from build123d import *

# Parameters (mm, degrees)
SKETCH1_W           = 12
SKETCH1_H           = 18.3
BOSS_EXTRUDE1_DEPTH = 3
SKETCH2_W           = 6
SKETCH2_H           = 18.3
BOSS_EXTRUDE2_DEPTH = 6
SKETCH3_R           = 1.575
CUT_EXTRUDE1_DEPTH  = 22.257704486
SKETCH4_W           = 6
SKETCH4_H           = 9
CUT_EXTRUDE2_DEPTH  = 6
FILLET1_R           = 3


with BuildPart() as part:
    # Sketch1 → Boss-Extrude1 (new body)
    with BuildSketch(Plane(origin=(0, 0, 0), x_dir=(1, 0, 0), z_dir=(0, 1, 0))):
        Rectangle(SKETCH1_W, SKETCH1_H)
    extrude(amount=BOSS_EXTRUDE1_DEPTH)

    # Sketch2 → Boss-Extrude2 (add)
    with BuildSketch(Plane(origin=(0, 3, 0), x_dir=(1, 0, 0), z_dir=(0, 1, 0))):
        with Locations((-3, 0)):
            Rectangle(SKETCH2_W, SKETCH2_H)
    extrude(amount=BOSS_EXTRUDE2_DEPTH)

    # Sketch3 → Cut-Extrude1 (cut, through all)
    with BuildSketch(Plane.XY.offset(9.15)):
        with Locations((-3, 6)):
            Circle(SKETCH3_R)
    extrude(amount=-CUT_EXTRUDE1_DEPTH, mode=Mode.SUBTRACT)

    # Sketch4 → Cut-Extrude2 (cut)
    with BuildSketch(Plane(origin=(0, 9, 0), x_dir=(1, 0, 0), z_dir=(0, 1, 0))):
        with Locations((-3, 0)):
            Rectangle(SKETCH4_W, SKETCH4_H)
    extrude(amount=-CUT_EXTRUDE2_DEPTH, mode=Mode.SUBTRACT)

    # Fillet1
    fillet1_edges = [part.edges().sort_by_distance(p)[0] for p in [
        (-6, 9, 6.825),
        (0, 9, 6.825),
        (-6, 9, -6.825),
        (0, 9, -6.825),
    ]]
    fillet(fillet1_edges, radius=FILLET1_R - 0.0001)  # a hair under: the kernel refuses the full size


solid = part.part
For this review, take the finished solid that the model builds, in its own axes (mm). A direction names the side the tool comes from. Round coordinates to 2 decimals unless told otherwise and drop trailing zeros. Write each loop counter-clockwise with the first axis right and the second up, starting at its lowest first coordinate (ties: lowest second). Pieces come first, ordered by that corner, then holes. Notation, with made-up numbers: (24, 15.5) - (31, 15.5) arc R31 cw to (31, 44.5) - close; hole circle Ø8 at (-6, 1.25). An arc over 180 degrees is marked (long way). Use a Markdown table: item, result.
Q1. Machinability: for faces 5 (the flat face through (-6, 2, 0)), 6 (the flat face through (0, 4, -7)), 7 (the flat face through (-1.7, 4.7, 4.5)), which of the approach directions +Z, -Z, +X, -X, +Y, -Y give a long, thin tool a straight path to every point of the face, cutting with its end or side? Answer none if there is none.
Derived:
| item | result |
|---|---|
| face 5 | +Z, -Z, -X, +Y, -Y |
| face 6 | +Z, -Z, +X, +Y |
| face 7 | +X, -X, +Y |
Q2. We need section A-A (y = 5.5). Give the boundary of the cut face in (x, z).
Derived:
| item | result |
|---|---|
| outline | (-6, -9.15) - (-4.49, -9.15) - (-4.49, -4.5) - (-6, -4.5) - close; (-6, 4.5) - (-4.49, 4.5) - (-4.49, 9.15) - (-6, 9.15) - close; (-1.51, -9.15) - (0, -9.15) - (0, -4.5) - (-1.51, -4.5) - close; (-1.51, 4.5) - (0, 4.5) - (0, 9.15) - (-1.51, 9.15) - close |
Q3. We need section D-D (z = -1.5). Give the boundary of the cut face in (x, y).
Derived:
| item | result |
|---|---|
| outline | (-6, 0) - (6, 0) - (6, 3) - (-6, 3) - close |
Q4. The part is to be moulded in two halves that separate along Z. For faces 1 (the flat face through (-1.7, 4.7, -4.5)), 2 (the flat face through (0, 4, 7)), 3 (the flat face through (-1, 3, 9.15)), 4 (the flat face through (-1, 3, -9.15)), say which applies: pulls with the +Z half, pulls with the -Z half, needs draft (parallel to the pull), parting line crosses it, or undercut.
Derived:
| item | result |
|---|---|
| face 1 | undercut |
| face 2 | needs draft |
| face 3 | pulls with the +Z half |
| face 4 | pulls with the -Z half |
Q5. Wall thickness on line 1 along Z through (x, y) = (-2, 8.5); line 2 along Y through (x, z) = (-3, 5.6) (3 decimals); line 3 along Y through (x, z) = (5, 3.75): over which ranges is each line inside the solid? List them lowest first.
Derived:
| item | result |
|---|---|
| line 1 | z = -9.15 to -4.5, 4.5 to 9.15 |
| line 2 | y = 0 to 4.425, 7.575 to 9 |
| line 3 | y = 0 to 3 |
Q6. We need section C-C (x = -3.25). Give the boundary of the cut face in (y, z), plus the area to 3 significant figures.
Derived:
| item | result |
|---|---|
| outline | (0, -9.15) - (4.44, -9.15) - (4.44, -4.5) - (3, -4.5) - (3, 4.5) - (4.44, 4.5) - (4.44, 9.15) - (0, 9.15) - close; (7.56, -9.15) - (8.99, -9.15) - (8.99, -4.5) - (7.56, -4.5) - close; (7.56, 4.5) - (8.99, 4.5) - (8.99, 9.15) - (7.56, 9.15) - close |
| area | 81.7 mm2 |
Q7. Clearance check with flat-ended pins moving along their axes: pin 1 (3.5 mm diameter, centred on y = 5, z = -7.5, fed in from +X); pin 2 (3 mm diameter, centred on x = -3, y = 6, fed in from +Z). State where each tip first meets the part, or that it passes through.
Derived:
| item | result |
|---|---|
| pin 1 | stops at x = 0 |
| pin 2 | passes through |
